from build123d import *

# Parameters (mm, degrees)
SKETCH_1_W                        = 1141
SKETCH_1_H                        = 151
SM_BASE_FLANGE_1_DEPTH            = 1
SM_EDGE_FLANGE_1_STRIP_W          = 5.4732
SM_EDGE_FLANGE_1_STRIP_H          = 1
SM_EDGE_FLANGE_1_STRIP_CUT_DEPTH  = 51
SM_EDGE_FLANGE_1_RELIEF_W         = 5.9732
SM_EDGE_FLANGE_1_RELIEF_H         = 0.5
SM_EDGE_FLANGE_1_RELIEF_CUT_DEPTH = 1
SM_EDGE_FLANGE_1_DEPTH            = 51
SM_EDGE_FLANGE_2_STRIP_W          = 5.4732
SM_EDGE_FLANGE_2_STRIP_H          = 1
SM_EDGE_FLANGE_2_STRIP_CUT_DEPTH  = 1041
SM_EDGE_FLANGE_2_RELIEF_W         = 5.9732
SM_EDGE_FLANGE_2_RELIEF_H         = 0.5
SM_EDGE_FLANGE_2_RELIEF_CUT_DEPTH = 1
SM_EDGE_FLANGE_2_DEPTH            = 1041
SM_EDGE_FLANGE_2_FLAT_DEPTH       = 1
SM_EDGE_FLANGE_4_STRIP_W          = 5.4732
SM_EDGE_FLANGE_4_STRIP_H          = 1
SM_EDGE_FLANGE_4_STRIP_CUT_DEPTH  = 51
SM_EDGE_FLANGE_4_RELIEF_W         = 5.9732
SM_EDGE_FLANGE_4_RELIEF_H         = 0.5
SM_EDGE_FLANGE_4_RELIEF_CUT_DEPTH = 1
SM_EDGE_FLANGE_4_DEPTH            = 51
SKETCH_15_R                       = 5
CUT_EXTRUDE_1_DEPTH               = 591.48391172
SKETCH_16_R                       = 3
CUT_EXTRUDE_2_DEPTH               = 576.7877213


# Sheet-metal steps are written as plain solids
with BuildPart() as part:
    # Sketch 1 → 基体-法兰1 (new body)
    with BuildSketch(Plane.XY):
        Rectangle(SKETCH_1_W, SKETCH_1_H)
    extrude(amount=-SM_BASE_FLANGE_1_DEPTH)

    # 边线-法兰1 strip (across the edge) → 边线-法兰1 strip cut (cut)
    with BuildSketch(Plane(origin=(570.5, 25.5, -1), x_dir=(-1, 0, 0), z_dir=(0, -1, 0))):
        with Locations((-1, -0.5)):
            Rectangle(SM_EDGE_FLANGE_1_STRIP_W, SM_EDGE_FLANGE_1_STRIP_H)
    extrude(amount=SM_EDGE_FLANGE_1_STRIP_CUT_DEPTH, mode=Mode.SUBTRACT)

    # 边线-法兰1 relief (on the sheet) → 边线-法兰1 relief cut (cut)
    with BuildSketch(Plane(origin=(568.7634, 25.5, -1), x_dir=(-1, 0, 0), z_dir=(0, 0, -1))):
        with Locations((-2.4866, 0.25)):
            Rectangle(SM_EDGE_FLANGE_1_RELIEF_W, SM_EDGE_FLANGE_1_RELIEF_H)
        with Locations((-2.4866, -51.25)):
            Rectangle(SM_EDGE_FLANGE_1_RELIEF_W, SM_EDGE_FLANGE_1_RELIEF_H)
    extrude(amount=-SM_EDGE_FLANGE_1_RELIEF_CUT_DEPTH, mode=Mode.SUBTRACT)

    # 边线-法兰1 section (across the edge) → 边线-法兰1 (add)
    with BuildSketch(Plane(origin=(570.5, 25.5, -1), x_dir=(-1, 0, 0), z_dir=(0, -1, 0))):
        with BuildLine():
            Line((0, 0.7366), (0, 19))
            Line((0, 19), (1, 19))
            Line((1, 19), (1, 0.7366))
            ThreePointArc((1, 0.7366), (1.215745145, 0.215745145), (1.7366, 0))
            Line((1.7366, 0), (1.7366, -1))
            ThreePointArc((1.7366, -1), (0.508638364, -0.491361636), (0, 0.7366))
        make_face()
    extrude(amount=SM_EDGE_FLANGE_1_DEPTH)

    # 边线-法兰2 strip (across the edge) → 边线-法兰2 strip cut (cut)
    with BuildSketch(Plane(origin=(-520.5, 75.5, -1), x_dir=(0, -1, 0), z_dir=(1, 0, 0))):
        with Locations((-1, -0.5)):
            Rectangle(SM_EDGE_FLANGE_2_STRIP_W, SM_EDGE_FLANGE_2_STRIP_H)
    sm_edge_flange_2_strip_cut = extrude(amount=SM_EDGE_FLANGE_2_STRIP_CUT_DEPTH, mode=Mode.SUBTRACT)

    # 边线-法兰2 relief (on the sheet) → 边线-法兰2 relief cut (cut)
    with BuildSketch(Plane(origin=(-520.5, 73.7634, -1), x_dir=(0, -1, 0), z_dir=(0, 0, -1))):
        with Locations((-2.4866, 0.25)):
            Rectangle(SM_EDGE_FLANGE_2_RELIEF_W, SM_EDGE_FLANGE_2_RELIEF_H)
        with Locations((-2.4866, -1041.25)):
            Rectangle(SM_EDGE_FLANGE_2_RELIEF_W, SM_EDGE_FLANGE_2_RELIEF_H)
    sm_edge_flange_2_relief_cut = extrude(amount=-SM_EDGE_FLANGE_2_RELIEF_CUT_DEPTH, mode=Mode.SUBTRACT)

    # 边线-法兰2 bend section (across the edge) → 边线-法兰2 (add)
    with BuildSketch(Plane(origin=(-520.5, 75.5, -1), x_dir=(0, -1, 0), z_dir=(1, 0, 0))):
        with BuildLine():
            Line((0, 0.7366), (1, 0.7366))
            ThreePointArc((1, 0.7366), (1.215745145, 0.215745145), (1.7366, 0))
            Line((1.7366, 0), (1.7366, -1))
            ThreePointArc((1.7366, -1), (0.508638364, -0.491361636), (0, 0.7366))
        make_face()
    sm_edge_flange_2 = extrude(amount=SM_EDGE_FLANGE_2_DEPTH)

    # 边线-法兰2 profile (on flange) → 边线-法兰2 flat (add)
    with BuildSketch(Plane(origin=(0, 75.5, -1), x_dir=(1, 0, 0), z_dir=(0, 1, 0))):
        Polygon((520.5, 0.7366), (520.5, 19), (257.5, 19), (257.5, 1), (241.5, 1), (241.5, 19), (-241.5, 19), (-241.5, 1), (-257.5, 1), (-257.5, 19), (-520.5, 19), (-520.5, 0.7366), align=None)
    sm_edge_flange_2_flat = extrude(amount=-SM_EDGE_FLANGE_2_FLAT_DEPTH)

    # 边线-法兰4 strip (across the edge) → 边线-法兰4 strip cut (cut)
    with BuildSketch(Plane(origin=(-570.5, -25.5, -1), x_dir=(1, 0, 0), z_dir=(0, 1, 0))):
        with Locations((-1, -0.5)):
            Rectangle(SM_EDGE_FLANGE_4_STRIP_W, SM_EDGE_FLANGE_4_STRIP_H)
    extrude(amount=SM_EDGE_FLANGE_4_STRIP_CUT_DEPTH, mode=Mode.SUBTRACT)

    # 边线-法兰4 relief (on the sheet) → 边线-法兰4 relief cut (cut)
    with BuildSketch(Plane(origin=(-568.7634, -25.5, -1), x_dir=(1, 0, 0), z_dir=(0, 0, -1))):
        with Locations((-2.4866, 0.25)):
            Rectangle(SM_EDGE_FLANGE_4_RELIEF_W, SM_EDGE_FLANGE_4_RELIEF_H)
        with Locations((-2.4866, -51.25)):
            Rectangle(SM_EDGE_FLANGE_4_RELIEF_W, SM_EDGE_FLANGE_4_RELIEF_H)
    extrude(amount=-SM_EDGE_FLANGE_4_RELIEF_CUT_DEPTH, mode=Mode.SUBTRACT)

    # 边线-法兰4 section (across the edge) → 边线-法兰4 (add)
    with BuildSketch(Plane(origin=(-570.5, -25.5, -1), x_dir=(1, 0, 0), z_dir=(0, 1, 0))):
        with BuildLine():
            Line((0, 0.7366), (0, 19))
            Line((0, 19), (1, 19))
            Line((1, 19), (1, 0.7366))
            ThreePointArc((1, 0.7366), (1.215745145, 0.215745145), (1.7366, 0))
            Line((1.7366, 0), (1.7366, -1))
            ThreePointArc((1.7366, -1), (0.508638364, -0.491361636), (0, 0.7366))
        make_face()
    extrude(amount=SM_EDGE_FLANGE_4_DEPTH)

    # 镜向1: 边线-法兰2 strip cut, 边线-法兰2 relief cut, 边线-法兰2, 边线-法兰2 flat across plane
    add(sm_edge_flange_2_strip_cut.mirror(Plane.ZX), mode=Mode.SUBTRACT)
    add(sm_edge_flange_2_relief_cut.mirror(Plane.ZX), mode=Mode.SUBTRACT)
    add(sm_edge_flange_2.mirror(Plane.ZX))
    add(sm_edge_flange_2_flat.mirror(Plane.ZX))

    # 草图15 → 切除-拉伸1 (cut, through all)
    with BuildSketch(Plane(origin=(0, 75.5, 0), x_dir=(1, 0, 0), z_dir=(0, 1, 0))):
        with Locations(Location((-228.5, 11, 0), (0, 0, 270))):
            Circle(SKETCH_15_R)
        with Locations(Location((228.5, 11, 0), (0, 0, 270))):
            Circle(SKETCH_15_R)
        with BuildLine():
            Line((-1.5, 16), (1.5, 16))
            ThreePointArc((1.5, 16), (6.5, 11), (1.5, 6))
            Line((1.5, 6), (-1.5, 6))
            ThreePointArc((-1.5, 6), (-6.5, 11), (-1.5, 16))
        make_face()
    extrude(amount=-CUT_EXTRUDE_1_DEPTH, mode=Mode.SUBTRACT)

    # 草图16 → 切除-拉伸2 (cut, through all)
    with BuildSketch(Plane(origin=(0, 0, -1), x_dir=(-1, 0, 0), z_dir=(0, 0, -1))):
        with Locations((-560.5, -66.5)):
            Circle(SKETCH_16_R)
        with Locations((-560.5, 65.5)):
            Circle(SKETCH_16_R)
        with Locations((561.5, -66.5)):
            Circle(SKETCH_16_R)
        with Locations((561.5, 65.5)):
            Circle(SKETCH_16_R)
    extrude(amount=-CUT_EXTRUDE_2_DEPTH, mode=Mode.SUBTRACT)


solid = part.part
The listing builds one solid part. Answer for the finished solid, in the listing's coordinates (mm). A direction names the side the tool comes from. Give positions to 0.01 mm unless a question says otherwise; leave off trailing zeros. Order: outer loops, then holes, each group sorted by start corner. A loop starts at its lowest first (then second) coordinate and runs counter-clockwise, first axis right, second up. Notation, with made-up numbers: (-35, 18.25) - (-5, 18.25) arc R25 ccw to (-5, 57.25) - close; hole circle Ø5 at (83, 58.25). An arc over 180 degrees is marked (long way). One line per item, written item: value. Start each with the question number.
1) A cutting plane is placed at B-B on y = -10. Give the vertices of the cut face in (x, z), then the cut area to 3 significant figures.
2) A tool of negligible diameter and unlimited length cuts with its end or side. For faces 1 (the face through (-7, -75.5, -11)), 2 (the face through (-7, -74.5, -11)), 3 (the face through (569.5, 0, -11)), from which of +Z, -Z, +X, -X, +Y, -Y can it reach the whole face along a straight path? Write none if from no direction.
3) Given pin 1 Ø0.7 at (y, z) = (74.5, -10) entering from -X; pin 2 Ø2 at (x, y) = (246, -10) entering from -Z; pin 3 Ø0.5 at (x, y) = (252, 75) entering from -Z, each flat-ended and moving along its own axis, determine where each tip first touches the part or whether it passes through.
4) The mould has two halves that part along X. Classify faces 4 (the face through (-569.5, 0, -11)), 5 (the face through (-8, 1, -1)), 6 (the face through (-570.5, 0, -11)), 7 (the face through (-8, 1, 0)): released by +X, released by -X, zero draft, split by the parting line, or undercut.
5) Find the intervals of material crossed by L1, parallel to Y at x = 560.5, z = -0.7; L2, parallel to X at y = 75.2, z = -11; L3, parallel to X at y = -2, z = -15, in increasing order.
6) A cutting plane is placed at A-A on x = 392.5. Give the vertices of the cut face in (y, z).
7) A cutting plane is placed at C-C on z = -11. State how many separate pieces and enclosed holes the cut face has, then the cut area to 3 significant figures.
Answer sheet:
1. outline: (-570.5, -20) - (-569.5, -20) - (-569.5, -1.74) arc R0.74 cw to (-568.76, -1) - (568.76, -1) arc R0.74 cw to (569.5, -1.74) - (569.5, -20) - (570.5, -20) - (570.5, -1.74) arc R1.74 ccw to (568.76, 0) - (-568.76, 0) arc R1.74 ccw to (-570.5, -1.74) - close
1. area: 1,180 mm2
2. face 1: +Z, -Z, +X, -X, -Y
2. face 2: -Z, +X, -X
2. face 3: -Z, +Y, -Y
3. pin 1: stops at x = -520.5
3. pin 2: stops at z = -1
3. pin 3: stops at z = -2
4. face 4: undercut
4. face 5: undercut
4. face 6: released by -X
4. face 7: zero draft
5. L1: y = -75.5 to -69.5, -63.5 to 62.5, 68.5 to 75.5
5. L2: x = -520.5 to -257.5, -241.5 to -233.5, -223.5 to -6.5, 6.5 to 223.5, 233.5 to 241.5, 257.5 to 520.5
5. L3: x = -570.5 to -569.5, 569.5 to 570.5
6. outline: (-75.5, -20) - (-74.5, -20) - (-74.5, -1.74) arc R0.74 cw to (-73.76, -1) - (73.76, -1) arc R0.74 cw to (74.5, -1.74) - (74.5, -20) - (75.5, -20) - (75.5, -1.74) arc R1.74 ccw to (73.76, 0) - (-73.76, 0) arc R1.74 ccw to (-75.5, -1.74) - close
7. separate pieces: 14
7. enclosed holes: 0
7. area: 2,050 mm2
